Autodesk Inventor part; units mm, degrees
ref_plane "YZ Plane" through (0, 0, 0) normal (1, 0, 0) x (0, 1, 0)
ref_plane "XZ Plane" through (0, 0, 0) normal (0, 1, 0) x (-1, 0, 0)
ref_plane "XY Plane" through (0, 0, 0) normal (0, 0, 1) x (1, 0, 0)
sketch "Sketch1" plane through (0, 0, 0) normal (0, 1, 0) x (-1, 0, 0)
  line L0 (5, 5) -> (-5, 5)
  line L1 (-5, 5) -> (-5, -5)
  line L2 (-5, -5) -> (5, -5)
  line L3 (5, -5) -> (5, 5)
  line L4 (5, 5) -> (-5, -5) construction
  line L5 (-5, 5) -> (5, -5) construction
  line L6 (15, 0) -> (15, -2)
  line L7 (15, -2) -> (5, -2)
  line L8 (5, -2) -> (5, 0)
  line L9 (15, 0) -> (15, 2)
  line L10 (15, 2) -> (5, 2)
  line L11 (-13, 13) -> (13, 13)
  line L12 (13, 13) -> (13, -13)
  line L13 (13, -13) -> (-13, -13)
  line L14 (-13, -13) -> (-13, 13)
  line L15 (-13, 13) -> (13, -13) construction
  line L16 (13, 13) -> (-13, -13) construction
  point P0 (0, 0)
  point P1 (10, 0)
  point P2 (13, 0)
  dimension "d0" = 10
  dimension "d1" = 10
  dimension "d2" = 10
  dimension "d3" = 2
  dimension "d4" = 5
  dimension "d5" = 2
  dimension "d6" = 3
  dimension "d7" = 3
extrude "Extrusion1" add sketch "Sketch1" along normal blind 38 contours L0 L1 L2 L3 L7 L12 L13 L14 L11 L10 | L10 L12 L7 L3
sketch "Sketch2" plane through (0, 0, 0) normal (1, 0, 0) x (0, 1, 0)
  line L0 (0, -13) -> (0, 13)
  line L1 (0, 5) -> (38, 5)
  line L2 (0, -5) -> (38, -5)
  line L3 (0, -13) -> (38, -13)
  circle A0 centre (4, 10) radius 1.75
  line L4 (-1.5, 15) -> (9.5, 15)
  line L5 (9.5, 15) -> (9.5, 5)
  line L6 (9.5, 5) -> (-1.5, 5)
  line L7 (-1.5, 5) -> (-1.5, 15)
  line L8 (-1.5, 15) -> (9.5, 5) construction
  line L9 (9.5, 15) -> (-1.5, 5) construction
  line L10 (0, 0) -> (20.9563, 0)
  circle A1 centre (14, 10) radius 1.75
  circle A2 centre (24, 10) radius 1.75
  line L11 (18.5, 15) -> (29.5, 15)
  line L12 (29.5, 15) -> (29.5, 5)
  line L13 (29.5, 5) -> (18.5, 5)
  line L14 (18.5, 5) -> (18.5, 15)
  line L15 (18.5, 15) -> (29.5, 5) construction
  line L16 (29.5, 15) -> (18.5, 5) construction
  circle A3 centre (4, -10) radius 1.75
  line L17 (-1.5, -15) -> (9.5, -15)
  line L18 (9.5, -15) -> (9.5, -5)
  line L19 (9.5, -5) -> (-1.5, -5)
  line L20 (-1.5, -5) -> (-1.5, -15)
  circle A4 centre (24, -10) radius 1.75
  line L21 (18.5, -15) -> (29.5, -15)
  line L22 (29.5, -15) -> (29.5, -5)
  line L23 (29.5, -5) -> (18.5, -5)
  line L24 (18.5, -5) -> (18.5, -15)
  line L25 (39, 2.5) -> (29, 2.5)
  line L26 (29, 2.5) -> (29, -2.5)
  line L27 (29, -2.5) -> (39, -2.5)
  line L28 (39, -2.5) -> (39, 2.5)
  line L29 (39, 2.5) -> (29, -2.5) construction
  line L30 (29, 2.5) -> (39, -2.5) construction
  line L31 (19, 2.5) -> (9, 2.5)
  line L32 (9, 2.5) -> (9, -2.5)
  line L33 (9, -2.5) -> (19, -2.5)
  line L34 (19, -2.5) -> (19, 2.5)
  line L35 (19, 2.5) -> (9, -2.5) construction
  line L36 (9, 2.5) -> (19, -2.5) construction
  line L37 (29, -2.5) -> (28.5, -2.5)
  line L38 (28.5, -2.5) -> (28.5, 2.5)
  line L39 (28.5, 2.5) -> (29, 2.5)
  line L40 (29, 2.5) -> (29, -2.5)
  line L41 (8.5, 2.75) -> (19.5, 2.75)
  line L42 (19.5, 2.75) -> (19.5, -2.75)
  line L43 (19.5, -2.75) -> (8.5, -2.75)
  line L44 (8.5, -2.75) -> (8.5, 2.75)
  line L45 (8.5, 2.75) -> (19.5, -2.75) construction
  line L46 (19.5, 2.75) -> (8.5, -2.75) construction
  line L47 (19, -2.5) -> (19.5, -2.5)
  line L48 (19, 2.5) -> (19.5, 2.5)
  line L49 (9, -2.5) -> (8.5, -2.5)
  line L50 (9, 2.5) -> (8.5, 2.5)
  point P0 (0, 0)
  point P1 (0, 0)
  point P2 (0, 10)
  point P3 (34, 10)
  point P4 (14, 0)
  point P5 (34, 0)
  point P6 (9.5, -13)
  point P7 (9.5, -5)
  point P8 (18.5, -5)
  point P9 (18.5, -13)
  point P10 (29.5, -13)
  point P11 (29.5, -5)
  point P12 (18.5, 5)
  point P13 (9, 0)
  point P14 (19, 0)
  dimension "d10" = 5
  dimension "d11" = 13
  dimension "d12" = 5
  dimension "d13" = 4
  dimension "d14" = 3.5
  dimension "d15" = 0
  dimension "d16" = 11
  dimension "d17" = 10
  dimension "d18" = 10
  dimension "d19" = 3.5
  dimension "d20" = 10
  dimension "d21" = 3.5
  dimension "d22" = 11
  dimension "d23" = 10
  dimension "d24" = 10
  dimension "d25" = 10
  dimension "d26" = 5
  dimension "d27" = 10
  dimension "d43" = 5
  dimension "d44" = 2.5
  dimension "d51" = 0.5
  dimension "d52" = 11
extrude "Extrusion2" cut sketch "Sketch2" along normal mid plane 5 contours L0 L2 L18 L3 | L14 L11 L12 L1 | L6 L7 L4 L5 L1 | L24 L2 L22 L3
extrude "Extrusion3" cut sketch "Sketch2" along normal mid plane 53 contours A0 | A2 | A3 | A4
extrude "Extrusion4" cut sketch "Sketch2" along normal mid plane 53 contours L32 L31 L34 L10 | L10 L34 L33 L32 | L28 L27 L26 L25
sketch "Sketch3" plane through (-5, 9, 2.5) normal (0, 0, -1) x (-1, 0, 0)
  line L0 (8, 10) -> (8, 0)
  line L1 (0, 0) -> (0, 10)
  line L2 (8, 10) -> (0, 10)
  line L3 (0, 20) -> (0, 29)
  line L4 (0, 20) -> (8, 20)
  circle A0 centre (5, 25) radius 1.75
  circle A1 centre (5, 5) radius 1.75
  line L5 (-7.5, 0.5) -> (-2.5, 0.5)
  line L6 (-5, 0.5) -> (-5, 17.2695)
  circle A2 centre (-15, 25) radius 1.75
  circle A3 centre (-15, 5) radius 1.75
  point P0 (-5, -9)
  dimension "d35" = 5
  dimension "d36" = 5
  dimension "d37" = 5
  dimension "d38" = 5
  dimension "d39" = 3.5
  dimension "d40" = 3.5
extrude "Extrusion5" cut sketch "Sketch3" along normal mid plane 53
sketch "Sketch4" plane through (0, 38, 0) normal (0, 1, 0) x (1, 0, 0)
  line L0 (6, -6) -> (-6, -6)
  line L1 (-6, -6) -> (-6, 6)
  line L2 (-6, 6) -> (6, 6)
  line L3 (6, 6) -> (6, -6)
  line L4 (6, -6) -> (-6, 6) construction
  line L5 (-6, -6) -> (6, 6) construction
  point P0 (0, 0)
  dimension "d45" = 12
  dimension "d46" = 12
extrude "Extrusion6" cut sketch "Sketch4" against normal blind 53
fillet "Fillet1" radius 2 4 edges at (-6, 19, -6) (6, 19, -6) (-6, 19, 6) (6, 19, 6)
extrude "Extrusion7" cut sketch "Sketch2" along normal mid plane 53 contours L44 L50 L32 L10 | L10 L32 L49 L44 | L34 L48 L42 L10 | L10 L42 L47 L34 | L26 L37 L38 L39
fillet "Fillet3" radius 0.74 24 edges at (-9.5, 28.5, -2.5) (9.5, 28.5, -2.5) (-9.5, 28.5, 2.5) (9.5, 28.5, 2.5) (-9.5, 19.5, -2.5) (9.5, 19.5, -2.5) (-9.5, 19.5, 2.5) (9.5, 19.5, 2.5) (-9.5, 8.5, -2.5) (9.5, 8.5, -2.5) (-9.5, 8.5, 2.5) (9.5, 8.5, 2.5) (2.5, 29.5, 9.5) (-2.5, 29.5, 9.5) (-2.5, 18.5, 9.5) (2.5, 18.5, 9.5) (2.5, 9.5, 9.5) (-2.5, 9.5, 9.5) (2.5, 29.5, -9.5) (-2.5, 29.5, -9.5) (-2.5, 18.5, -9.5) (2.5, 18.5, -9.5) (-2.5, 9.5, -9.5) (2.5, 9.5, -9.5)
sketch "Sketch5" plane through (-13, 0, -13) normal (-1, 0, 0) x (0, 0, 1)
  point P0 (13, 0)
equation "\"d44\" = 0.5 * d43"
properties part number "carriage_v1" material "ABS プラスチック"
Verification items for the finished model (mm, model axes). A direction names the side the tool comes from. Give positions to 0.01 mm unless a question says otherwise; leave off trailing zeros. Order: outer loops, then holes, each group sorted by start corner. A loop starts at its lowest first (then second) coordinate and runs counter-clockwise, first axis right, second up. Notation, with made-up numbers: (68, -0.75) -> (123, -0.75) arc R22 cw to (123, 24.25) -> close; hole circle Ø9 at (39.5, 54.5). An arc over 180 degrees is marked (long way). One line per item, written item: value.
(1) Sectioned sample at D-D on z = -10. Count the separate pieces of the cut face and the enclosed holes in it, then the cut area to 3 significant figures.
Final values:
separate pieces: 4
enclosed holes: 4
area: 701 mm^2
(2) Tool access check on faces 1 (the face through (0, 29.5, 10)), 2 (the face through (-8, 34, 2.5)), 3 (the face through (-2.5, 4, -8)), 4 (the face through (-5.4, 18.73, 5.43)), 5 (the face through (-10, 19.5, 0)). Record the directions out of +Z, -Z, +X, -X, +Y, -Y that give a thin tool (end or side, any length) a straight path to the whole face; none if there is none.
Final values:
face 1: +Z, -Z
face 2: +X, -X, +Y
face 3: +Z, -Z, -Y
face 4: +Y, -Y
face 5: +X, -X
(3) Sectioned sample at C-C on x = -0.25. Record the cut outline in (y, z).
Final values:
outline: (9.5, -13) -> (18.5, -13) -> (18.5, -6) -> (9.5, -6) -> close; (9.5, 6) -> (18.5, 6) -> (18.5, 13) -> (9.5, 13) -> close; (29.5, -13) -> (38, -13) -> (38, -6) -> (29.5, -6) -> close; (29.5, 6) -> (38, 6) -> (38, 13) -> (29.5, 13) -> close
(4) Scan lines: line 1 along Z through (x, y) = (10.5, 4); line 2 along Y through (x, z) = (10, 10); line 3 along Y through (x, z) = (7.25, 10). Record each from-to range of solid material in increasing order. Write a range as [from, to].
Final values:
line 1: [-13, -11.75], [-8.25, 8.25], [11.75, 13]
line 2: [0, 2.25], [5.75, 12.25], [15.75, 22.25], [25.75, 32.25], [35.75, 38]
line 3: [0, 2.25], [5.75, 22.25], [25.75, 38]
(5) Sectioned sample at A-A on x = 3.25. Record the cut outline in (y, z).
Final values:
outline: (0, -13) -> (38, -13) -> (38, -6) -> (0, -6) -> close; (0, 6) -> (38, 6) -> (38, 13) -> (0, 13) -> close; hole circle Ø3.5 at (4, -10); hole circle Ø3.5 at (4, 10); hole circle Ø3.5 at (24, -10); hole circle Ø3.5 at (24, 10)
(6) Sectioned sample at B-B on z = -1. Record the cut outline in (x, y).
Final values:
outline: (-13, 0) -> (-6, 0) -> (-6, 8.5) -> (-13, 8.5) -> close; (-13, 19.5) -> (-6, 19.5) -> (-6, 28.5) -> (-13, 28.5) -> close; (6, 0) -> (13, 0) -> (13, 8.5) -> (6, 8.5) -> close; (6, 19.5) -> (13, 19.5) -> (13, 28.5) -> (6, 28.5) -> close
(7) Draft check along Z on faces 6 (the face through (3, 19, 13)), 7 (the face through (-3, 19, -13)), 8 (the face through (0, 29.5, -10)), 9 (the face through (8, 14, -2.5)). Enter one of: pulls with the +Z half, pulls with the -Z half, needs draft (parallel to the pull), parting line crosses it, or undercut.
Final values:
face 6: pulls with the +Z half
face 7: pulls with the -Z half
face 8: needs draft
face 9: undercut
(8) Gauge pin test, flat ends, axial feed: pin 1 (3.5 mm diameter, centred on x = -8.5, y = 34.5, fed in from +Z); pin 2 (1.8 mm diameter, centred on x = 0.5, z = 11, fed in from -Y); pin 3 (1.8 mm diameter, centred on x = -11, z = -0.5, fed in from +Y). Record the tip position at first contact, or that the pin passes through.
Final values:
pin 1: z = 13
pin 2: y = 9.5
pin 3: y = 28.5
